```python
from build123d import *

# Parameters (mm, degrees)
EXTRUDE_1_DEPTH     = 36.5
CUT_EXTRUDE_1_DEPTH = 39.585575484
SKETCH_3_W          = 8.80936978
SKETCH_3_H          = 5.154088086
EXTRUDE_3_DEPTH     = 8.25
SKETCH_4_R          = 0.95
CUT_EXTRUDE_2_DEPTH = 10
SKETCH_5_W          = 4
SKETCH_5_H          = 3.5
SKETCH_6_R          = 0.8
CUT_EXTRUDE_3_DEPTH = 38.904707278


with BuildPart() as part:
    # ｽｹｯﾁ1 → ﾎﾞｽ - 押し出し1 (new body)
    with BuildSketch(Plane.XY):
        Polygon((-3.49531511, 0), (-1.50468489, 0), (-0.99531511, -1.2), (0.99531511, -1.2), (1.50468489, 0), (3.49531511, 0), (4.00468489, -1.2), (4.90468489, -1.2), (4.90468489, 4), (3.146705018, 7.77), (-3.146705018, 7.77), (-4.90468489, 4), (-4.90468489, -1.2), (-4.00468489, -1.2), align=None)
    extrude(amount=EXTRUDE_1_DEPTH)

    # ｽｹｯﾁ2 → ｶｯﾄ - 押し出し1 (cut, through all)
    with BuildSketch(Plane(origin=(4.90468489, 0, 0), x_dir=(0, 0, -1), z_dir=(1, 0, 0))):
        Polygon((-36.5, 4), (-34.742020129, 7.77), (-36.5, 7.77), align=None)
        Polygon((-1.757979871, 7.77), (0, 7.77), (0, 4), align=None)
    extrude(amount=-CUT_EXTRUDE_1_DEPTH, mode=Mode.SUBTRACT)

    # 面取り1
    # the kernel refuses this chamfer: 0.5 mm, written as the material it takes off along each edge
    with BuildSketch(Plane(origin=(-2.939971721, 7.467897404, 1.964713169), x_dir=(0.19590671622030337, 0.5268881046463144, 0.8270486586180961), z_dir=(-0.41632572739388213, 0.8082980746110389, -0.4163257273938791)), Plane(origin=(2.939971721, 7.467897404, 1.964713169), x_dir=(-0.8270486586180947, 0.5268881046463163, 0.1959067162203037), z_dir=(0.4163257273938816, 0.8082980746110384, -0.41632572739388035))) as chamfer_1_piece_1:
        Polygon((-0.400884159, 0.228990916), (0.459173014, 0.228990916), (-0.058288855, -0.457981831), align=None)
    extrude(amount=0.4579583, mode=Mode.SUBTRACT)
    with BuildSketch(Plane(origin=(-2.939971721, 7.467897404, 34.535286831), x_dir=(-0.1959067162203061, -0.5268881046463181, 0.827048658618093), z_dir=(-0.4163257273938827, 0.8082980746110371, 0.4163257273938816))) as chamfer_1_piece_2:
        Polygon((-0.459173014, 0.228990916), (0.400884159, 0.228990916), (0.058288855, -0.457981831), align=None)
    extrude(amount=0.4579583, mode=Mode.SUBTRACT)
    with BuildSketch(Plane(origin=(2.939971721, 7.467897404, 34.535286831), x_dir=(-0.8270486586180942, 0.5268881046463159, -0.19590671622030717), z_dir=(0.41632572739387785, 0.8082980746110375, 0.41632572739388596))) as chamfer_1_piece_3:
        Polygon((-0.400884159, -0.228990916), (0.459173014, -0.228990916), (-0.058288855, 0.457981831), align=None)
    extrude(amount=0.4579583, mode=Mode.SUBTRACT)
    with BuildSketch(Plane(origin=(4.90468489, -2.485841494, 36.5), x_dir=(-0.999621916911297, 0, 0.0274958766105822), z_dir=(0, 1, 0)), Plane(origin=(-4.90468489, 5.285841494, 36.5), x_dir=(0.999621916911297, 0, 0.0274958766105822), z_dir=(0, -1, 0))) as chamfer_1_piece_4:
        with BuildLine():
            Line((0.514336598, 0), (-0.028273577, -0.513558897))
            Line((-0.028273577, -0.513558897), (-0.038269797, -0.513283938))
            ThreePointArc((-0.038269797, -0.513283938), (-0.017064614, -0.256698915), (-0.009996219, 0.000274959))
            Line((-0.009996219, 0.000274959), (0.000274959, 0.009996219))
            ThreePointArc((0.000274959, 0.009996219), (0.257248832, 0.002927825), (0.514611556, 0.009996219))
            Line((0.514611556, 0.009996219), (0.514336598, 0))
        make_face()
    extrude(amount=7.771682988, mode=Mode.SUBTRACT)
    with BuildSketch(Plane(origin=(-4.90468489, 5.285841494, 0), x_dir=(0.9996219169112968, 0, -0.02749587661058639), z_dir=(0, -1, 0)), Plane(origin=(4.90468489, -2.485841494, 0), x_dir=(-0.9996219169112968, 0, -0.02749587661058639), z_dir=(0, 1, 0))) as chamfer_1_piece_5:
        with BuildLine():
            Line((0.514336598, 0), (-0.028273577, 0.513558897))
            Line((-0.028273577, 0.513558897), (-0.038269797, 0.513283938))
            ThreePointArc((-0.038269797, 0.513283938), (-0.017064614, 0.256698915), (-0.009996219, -0.000274959))
            Line((-0.009996219, -0.000274959), (0.000274959, -0.009996219))
            ThreePointArc((0.000274959, -0.009996219), (0.257248832, -0.002927825), (0.514611556, -0.009996219))
            Line((0.514611556, -0.009996219), (0.514336598, 0))
        make_face()
    extrude(amount=7.771682988, mode=Mode.SUBTRACT)
    with BuildSketch(Plane(origin=(-3.146705018, 7.77, 0.46553106), x_dir=(-0.4413655645980938, -0.8973273864019787, 0), z_dir=(0, 0, 1))) as chamfer_1_piece_6:
        with BuildLine():
            Line((0.516979525, 0), (-0.237770334, 0.459056747))
            Line((-0.237770334, 0.459056747), (-0.246743608, 0.454643091))
            ThreePointArc((-0.246743608, 0.454643091), (-0.123037104, 0.227486173), (-0.008973274, -0.004413656))
            Line((-0.008973274, -0.004413656), (0.000207861, -0.009997839))
            ThreePointArc((0.000207861, -0.009997839), (0.25858594, -0.004626004), (0.517187386, -0.009997839))
            Line((0.517187386, -0.009997839), (0.516979525, 0))
        make_face()
    extrude(amount=35.568937881, mode=Mode.SUBTRACT)
    with BuildSketch(Plane(origin=(3.146705018, 7.77, 0.46553106), x_dir=(0.4413655645980931, -0.8973273864019791, 0), z_dir=(0, 0, 1))) as chamfer_1_piece_7:
        with BuildLine():
            Line((0.516979525, 0), (-0.237770334, -0.459056747))
            Line((-0.237770334, -0.459056747), (-0.246743608, -0.454643091))
            ThreePointArc((-0.246743608, -0.454643091), (-0.123037104, -0.227486173), (-0.008973274, 0.004413656))
            Line((-0.008973274, 0.004413656), (0.000207861, 0.009997839))
            ThreePointArc((0.000207861, 0.009997839), (0.25858594, 0.004626004), (0.517187386, 0.009997839))
            Line((0.517187386, 0.009997839), (0.516979525, 0))
        make_face()
    extrude(amount=35.568937881, mode=Mode.SUBTRACT)
    with BuildSketch(Plane(origin=(4.43915383, 7.77, 34.742020129), x_dir=(0, -0.8973273864019841, 0.4413655645980827), z_dir=(-1, 0, 0))) as chamfer_1_piece_8:
        with BuildLine():
            Line((0.516979525, 0), (-0.237770334, -0.459056747))
            Line((-0.237770334, -0.459056747), (-0.246743608, -0.454643091))
            ThreePointArc((-0.246743608, -0.454643091), (-0.123037104, -0.227486173), (-0.008973274, 0.004413656))
            Line((-0.008973274, 0.004413656), (0.000207861, 0.009997839))
            ThreePointArc((0.000207861, 0.009997839), (0.25858594, 0.004626004), (0.517187386, 0.009997839))
            Line((0.517187386, 0.009997839), (0.516979525, 0))
        make_face()
    extrude(amount=8.87830766, mode=Mode.SUBTRACT)
    with BuildSketch(Plane(origin=(2.645006091, 8.845896822, 34.240321201), x_dir=(-0.9208340423276122, -0.3421923931836881, 0.1870000869994703), z_dir=(0.38928162063502675, -0.8348171294789896, 0.3892816206350195)), Plane(origin=(-5.406383817, 2.924103178, 37.001698928), x_dir=(0.9208340423276125, -0.34219239318369504, 0.18700008699945572), z_dir=(0.38928162063502675, 0.8348171294789896, -0.3892816206350195))) as chamfer_1_piece_9:
        with BuildLine():
            Line((0.515512576, 0), (-0.117174183, 0.502019349))
            Line((-0.117174183, 0.502019349), (-0.126965941, 0.499989208))
            ThreePointArc((-0.126965941, 0.499989208), (-0.062103739, 0.250280562), (-0.009791758, -0.002030141))
            Line((-0.009791758, -0.002030141), (0.000248629, -0.009996909))
            ThreePointArc((0.000248629, -0.009996909), (0.257845581, -0.003590326), (0.515761205, -0.009996909))
            Line((0.515761205, -0.009996909), (0.515512576, 0))
        make_face()
    extrude(amount=7.093521964, mode=Mode.SUBTRACT)
    with BuildSketch(Plane(origin=(2.645006091, 8.845896822, 2.259678799), x_dir=(-0.9208340423276122, -0.3421923931836898, -0.18700008699946685), z_dir=(0.3892816206350268, -0.8348171294789898, -0.3892816206350187)), Plane(origin=(-5.406383817, 2.924103178, -0.501698928), x_dir=(0.9208340423276122, -0.34219239318368977, -0.1870000869994671), z_dir=(0.3892816206350268, 0.8348171294789898, 0.3892816206350187))) as chamfer_1_piece_10:
        with BuildLine():
            Line((0.515512576, 0), (-0.117174183, -0.502019349))
            Line((-0.117174183, -0.502019349), (-0.126965941, -0.499989208))
            ThreePointArc((-0.126965941, -0.499989208), (-0.062103739, -0.250280562), (-0.009791758, 0.002030141))
            Line((-0.009791758, 0.002030141), (0.000248629, 0.009996909))
            ThreePointArc((0.000248629, 0.009996909), (0.257845581, 0.003590326), (0.515761205, 0.009996909))
            Line((0.515761205, 0.009996909), (0.515512576, 0))
        make_face()
    extrude(amount=7.093521964, mode=Mode.SUBTRACT)
    with BuildSketch(Plane(origin=(4.43915383, 7.77, 1.757979871), x_dir=(0, -0.8973273864019825, -0.4413655645980858), z_dir=(-1, 0, 0))) as chamfer_1_piece_11:
        with BuildLine():
            Line((0.516979525, 0), (-0.237770334, 0.459056747))
            Line((-0.237770334, 0.459056747), (-0.246743608, 0.454643091))
            ThreePointArc((-0.246743608, 0.454643091), (-0.123037104, 0.227486173), (-0.008973274, -0.004413656))
            Line((-0.008973274, -0.004413656), (0.000207861, -0.009997839))
            ThreePointArc((0.000207861, -0.009997839), (0.25858594, -0.004626004), (0.517187386, -0.009997839))
            Line((0.517187386, -0.009997839), (0.516979525, 0))
        make_face()
    extrude(amount=8.87830766, mode=Mode.SUBTRACT)

    # ｽｹｯﾁ3 → ﾎﾞｽ - 押し出し3 (add)
    with BuildSketch(Plane.XY.offset(36.5)):
        with Locations((0, 1.377044043)):
            Rectangle(SKETCH_3_W, SKETCH_3_H)
    extrude_3 = extrude(amount=-EXTRUDE_3_DEPTH)

    # ｽｹｯﾁ4 → ｶｯﾄ - 押し出し2 (cut)
    with BuildSketch(Plane.XY.offset(36.5)):
        with Locations((0, 0.6)):
            Circle(SKETCH_4_R)
    cut_extrude_2 = extrude(amount=-CUT_EXTRUDE_2_DEPTH, mode=Mode.SUBTRACT)

    # ﾐﾗｰ1: ﾎﾞｽ - 押し出し3, ｶｯﾄ - 押し出し2 across plane
    add(extrude_3.mirror(Plane(origin=(0, 0, 18.25), x_dir=(1, 0, 0), z_dir=(0, 0, -1))))
    add(cut_extrude_2.mirror(Plane(origin=(0, 0, 18.25), x_dir=(1, 0, 0), z_dir=(0, 0, -1))), mode=Mode.SUBTRACT)

    # ｽｹｯﾁ5 → ｶｯﾄ - 回転1 (revolve, cut)
    with BuildSketch(Plane(origin=(0, 0.6, 0), x_dir=(1, 0, 0), z_dir=(0, 1, 0))):
        with Locations((2, -33.25)):
            Rectangle(SKETCH_5_W, SKETCH_5_H)
        with Locations((2, -3.25)):
            Rectangle(SKETCH_5_W, SKETCH_5_H)
    revolve(axis=Axis((0, 0.6, 26.5), (0, 0, 1)), mode=Mode.SUBTRACT)

    # ｽｹｯﾁ6 → ｶｯﾄ - 押し出し3 (cut, through all)
    with BuildSketch(Plane(origin=(0, 7.77, 0), x_dir=(1, 0, 0), z_dir=(0, 1, 0))):
        with Locations(Location((0, -18.25, 0), (0, 0, 270))):
            Circle(SKETCH_6_R)
    extrude(amount=-CUT_EXTRUDE_3_DEPTH, mode=Mode.SUBTRACT)


solid = part.part
```
Could you check a few things on this model? Use its own coordinates, in mm. A direction names the side the tool comes from. Round coordinates to 2 decimals unless told otherwise and drop trailing zeros. Loops run counter-clockwise (first coordinate to the right, second up) from the corner with the lowest first, then second, coordinate; pieces in that order, holes last. Notation, with made-up numbers: M 12,-7.75 L 57,-7.75 A14 cw 57,5.25 Z; hole C -37,-24.5 d4. An arc over 180 degrees is marked long. Write item = value, one per line.
1. Thinking about a two-plate mould opening in X: for faces 1 (the face through (0, 2, 35)), 2 (the face through (4.14, 5.64, 18)), 3 (the face through (0, 2, 36.5)), which applies, +X half, -X half, draft (parallel to the pull), parting line (faces both ways), or undercut?
Results below:
face_1 = undercut
face_2 = +X half
face_3 = draft
2. I want a section at C-C, the plane z = 29. Write out the boundary of the cut face in (x, y), and give its area (3 significant figures).
Results below:
outline = M -4.9,-1.2 L 4.9,-1.2 L 4.9,4 L 3.36,7.32 L 2.65,7.77 L -2.65,7.77 L -3.36,7.32 L -4.9,4 Z; hole C 0,0.6 d1.9
area = 78.3 mm²
3. I want a section at D-D, the plane y = 3.5. Write out the boundary of the cut face in (x, z) (3 decimals).
Results below:
outline = M -4.905,0.5 L -4.405,0 L 4.405,0 L 4.905,0.5 L 4.905,36 L 4.405,36.5 L -4.405,36.5 L -4.905,36 Z; hole M -2.755,1.5 L 2.755,1.5 L 2.755,5 L -2.755,5 Z; hole M -2.755,31.5 L 2.755,31.5 L 2.755,35 L -2.755,35 Z; hole C 0,18.25 d1.6
4. Will these pins go through, and if not, where does the flat tip stop? P1, Ø3, axis at x = 0, y = 0.6, coming from the -Z side; P2, Ø2, axis at x = 1, y = 5.5, coming from the +Z side; P3, Ø1.5, axis at x = 0, y = 0.5, coming from the -Z side; P4, Ø1.1, axis at x = 0, y = 0.6, coming from the +Z side.
Results below:
P1 = 0
P2 = 36.27
P3 = 10
P4 = 26.5
5. I need wall thicknesses on probe 1 along Z at (x, y) = (3.25, -1); probe 2 along Z at (x, y) = (1.25, 2.75); probe 3 along X at (y, z) = (0.6, 6.3). Which ranges of each line are inside material? Lowest first, please.
Results below:
probe_1 = 0 to 1.5, 5 to 8.25, 28.25 to 31.5, 35 to 36.5
probe_2 = 0 to 1.5, 5 to 31.5, 35 to 36.5
probe_3 = -4.9 to -0.95, 0.95 to 4.9
6. I want a section at B-B, the plane z = 18.25. Write out the boundary of the cut face in (x, y), and give its area (3 significant figures).
Results below:
outline = M -4.9,-1.2 L -4,-1.2 L -3.5,0 L -1.5,0 L -1,-1.2 L -0.8,-1.2 L -0.8,7.77 L -2.65,7.77 L -3.36,7.32 L -4.9,4 Z; M 0.8,-1.2 L 1,-1.2 L 1.5,0 L 3.5,0 L 4,-1.2 L 4.9,-1.2 L 4.9,4 L 3.36,7.32 L 2.65,7.77 L 0.8,7.77 Z
area = 60.8 mm²
7. Which directions (+Z, -Z, +X, -X, +Y, -Y) give clear straight access to the entire face, cutting with the end or side of a thin tool? Please do faces 4 (the face through (1.246, -0.608, 18.11)), 5 (the face through (0, 1, 10)), 6 (the face through (0.1, 4.6, 33.2)), 7 (the face through (3.856, 5.659, 35.459)).
Results below:
face_4 = -Y
face_5 = -Z
face_6 = none
face_7 = +Z, +X, +Y
